Verification items for this drawing (mm, ordinates from the low corner). Give positions to 0.01 mm unless a question says otherwise; leave off trailing zeros. Loops run counter-clockwise (first coordinate to the right, second up) from the corner with the lowest first, then second, coordinate; pieces in that order, holes last. Notation, with made-up numbers: (35, 49) -> (91, 49) arc R28 ccw to (91, 78) -> close; hole circle Ø8 at (14, 48.25). An arc over 180 degrees is marked (long way). Answer as a JSON object with one key per item and string values.
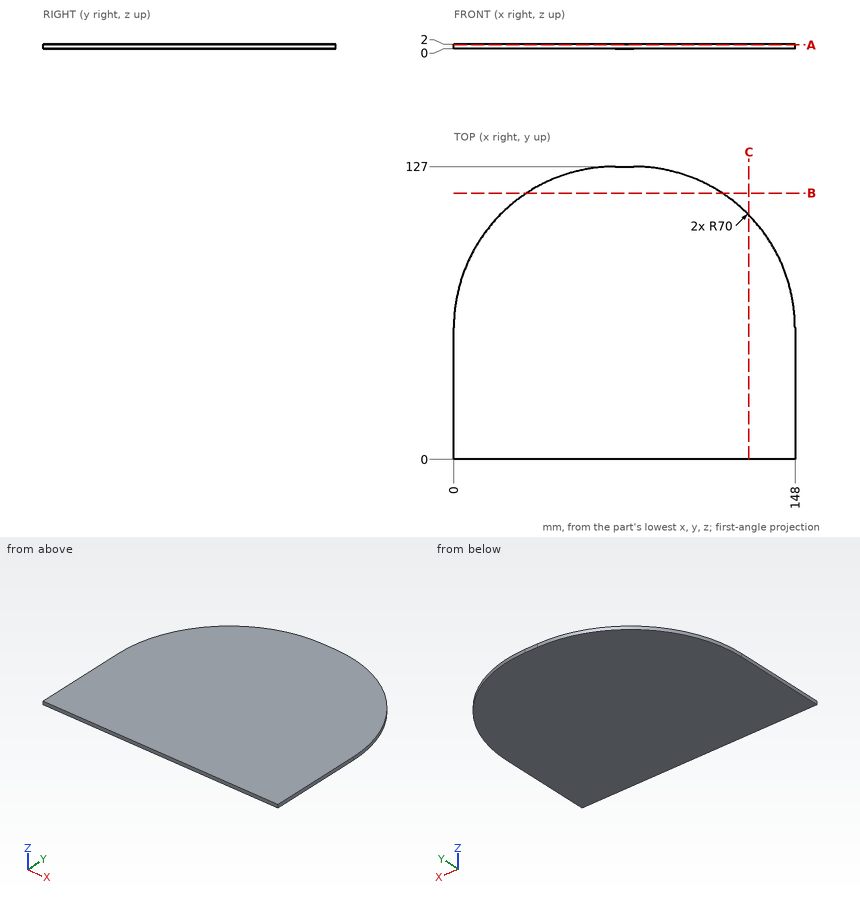
1) Depth check by flat-ended pin: P1, Ø1.5, axis at x = 63.5, y = 33.5, coming from the -Z side. Enter the tip coordinate at first touch or a pass-through.
Geometry check:
{"P1": "stops at z = 0"}
2) Material ranges on line 1 along Y through (x, z) = (68.5, 1.35); line 2 along Y through (x, z) = (123.5, 1.45); line 3 along X through (y, z) = (107, 0.4), recorded low to high. Write a range as from..to.
Geometry check:
{"line 1": "y = 0..126.98", "line 2": "y = 0..110.2", "line 3": "x = 21.01..126.99"}
3) Section check B-B on y = 115.5. Record the cut outline in (x, z).
Geometry check:
{"outline": "(31.56, 0) -> (116.44, 0) -> (116.44, 2) -> (31.56, 2) -> close"}
4) Section check A-A on z = 1.65. Record the cut outline in (x, y).
Geometry check:
{"outline": "(0, 0) -> (148, 0) -> (148, 57) arc R70 ccw to (78, 127) -> (70, 127) arc R70 ccw to (0, 57) -> close"}
5) Section check C-C on x = 128. Record the cut outline in (y, z), plus the area to 3 significant figures.
Geometry check:
{"outline": "(0, 0) -> (105.99, 0) -> (105.99, 2) -> (0, 2) -> close", "area": "212 mm2"}
